Input: part model. Units: mm. Frame: model coordinates. Coordinates: 2 decimals unless noted, no trailing zeros. Loops run counter-clockwise (first coordinate to the right, second up) from the corner with the lowest first, then second, coordinate; pieces in that order, holes last. Notation, with made-up numbers: (16.25, -15.5) - (26.25, -15.5) arc R21 cw to (26.25, 15.5) - close; hole circle Ø11 at (-15, -26.75). An arc over 180 degrees is marked (long way). Use a Markdown table: item, result. Add a question column.
1. Section query D-D on x = 40. Return the cut outline in (y, z), then the cut area to 3 significant figures.
2. Section query A-A on z = 12.25. Return the cut outline in (x, y), then the cut area to 3 significant figures.
3. Ray query, L1, parallel to X at y = 1, z = 11.5; L2, parallel to X at y = 0.8, z = 4; L3, parallel to X at y = 0.85, z = 6.5. Return the intervals inside material, ascending. Write a range as [from, to].
4. Contact query for a flat-ended pin moving along its axis: P1, Ø1, axis at x = 44.5, z = 7, coming from the +Y side. Output: stop coordinate, or through.
5. Draft query along X for faces 1 (the face through (30, 0, 8)), 2 (the face through (23.2, 1.5, 7.5)), 3 (the face through (46.4, 1.5, 7.5)), 4 (the face through (-4.866, 2, 9)). Return one class per face: released by +X, released by -X, zero draft, split by the parting line, or undercut.
6. Section query C-C on z = 4. Return the cut outline in (x, y), then the cut area to 3 significant figures.
7. Section query B-B on y = 2. Return the cut outline in (x, z) (3 decimals), then the cut area to 3 significant figures.
```python
from build123d import *

# Parameters (mm, degrees)
BOSS_EXTRUDE1_DEPTH = 3
SKETCH2_W           = 75.494873271
SKETCH2_H           = 16.574066579
CUT_EXTRUDE1_DEPTH  = 3
FILLET1_R           = 0.5


with BuildPart() as part:
    # Sketch1 → Boss-Extrude1 (new body)
    with BuildSketch(Plane(origin=(0, 0, 0), x_dir=(1, 0, 0), z_dir=(0, 1, 0))):
        with BuildLine():
            ThreePointArc((51.666035076, -4.495071474), (57.875, -2.537392354), (64.083964924, -4.495071474))
            Line((64.083964924, -4.495071474), (64.083964924, -11.181167218))
            ThreePointArc((64.083964924, -11.181167218), (57.875, -9.223488098), (51.666035076, -11.181167218))
            ThreePointArc((51.666035076, -11.181167218), (46.3, -13.686095744), (40.933964924, -11.181167218))
            ThreePointArc((40.933964924, -11.181167218), (34.725, -9.223488098), (28.516035077, -11.181167218))
            ThreePointArc((28.516035077, -11.181167218), (23.15, -13.686095744), (17.783964924, -11.181167218))
            ThreePointArc((17.783964924, -11.181167218), (11.575, -9.223488098), (5.366035077, -11.181167218))
            ThreePointArc((5.366035077, -11.181167218), (0, -13.686095744), (-5.366035076, -11.181167218))
            Line((-5.366035076, -11.181167218), (-5.366035076, -4.495071474))
            ThreePointArc((-5.366035076, -4.495071474), (0, -7), (5.366035076, -4.495071474))
            ThreePointArc((5.366035076, -4.495071474), (11.575, -2.537392354), (17.783964924, -4.495071474))
            ThreePointArc((17.783964924, -4.495071474), (23.15, -7), (28.516035076, -4.495071474))
            ThreePointArc((28.516035076, -4.495071474), (34.725, -2.537392354), (40.933964924, -4.495071474))
            ThreePointArc((40.933964924, -4.495071474), (46.3, -7), (51.666035076, -4.495071474))
        make_face()
    extrude(amount=BOSS_EXTRUDE1_DEPTH)

    # Sketch2 → Cut-Extrude1 (cut)
    with BuildSketch(Plane(origin=(0, 3, 0), x_dir=(1, 0, 0), z_dir=(0, 1, 0))):
        with Locations((29.270514079, -6.984979931)):
            Rectangle(SKETCH2_W, SKETCH2_H)
        with BuildLine():
            Line((63.583964924, -10.267724094), (63.583964924, -4.759291488))
            ThreePointArc((63.583964924, -4.759291488), (57.778030808, -3.037847716), (52.005454008, -4.868038061))
            ThreePointArc((52.005454008, -4.868038061), (46.3, -7.5), (40.594545992, -4.868038061))
            ThreePointArc((40.594545992, -4.868038061), (34.725, -3.037392354), (28.855454008, -4.868038061))
            ThreePointArc((28.855454008, -4.868038061), (23.15, -7.5), (17.444545992, -4.868038061))
            ThreePointArc((17.444545992, -4.868038061), (11.575, -3.037392354), (5.705454008, -4.868038061))
            ThreePointArc((5.705454008, -4.868038061), (0.593454673, -7.476483903), (-4.866035076, -5.707162398))
            Line((-4.866035076, -5.707162398), (-4.866035076, -10.995585579))
            ThreePointArc((-4.866035076, -10.995585579), (0.121449449, -13.184961032), (5.023650974, -10.810769172))
            ThreePointArc((5.023650974, -10.810769172), (11.575, -8.723488098), (18.126349026, -10.810769172))
            ThreePointArc((18.126349026, -10.810769172), (23.15, -13.186095744), (28.173650974, -10.810769172))
            ThreePointArc((28.173650974, -10.810769172), (34.725, -8.723488098), (41.276349026, -10.810769172))
            ThreePointArc((41.276349026, -10.810769172), (46.3, -13.186095744), (51.323650974, -10.810769172))
            ThreePointArc((51.323650974, -10.810769172), (57.373874034, -8.734580825), (63.583964924, -10.267724094))
        make_face(mode=Mode.SUBTRACT)
    extrude(amount=-CUT_EXTRUDE1_DEPTH, mode=Mode.SUBTRACT)

    # Fillet1
    fillet1_edges = [part.edges().sort_by_distance(p)[0] for p in [
        (63.583964924, 1.5, 10.267724094),
        (63.583964924, 1.5, 4.759291488),
        (-4.866035076, 1.5, 5.707162398),
        (-4.866035076, 1.5, 10.995585579),
    ]]
    fillet(fillet1_edges, radius=FILLET1_R)


solid = part.part
```
Resolved:
| question | item | result |
|---|---|---|
| 1 | outline | (0, 4.49) - (3, 4.49) - (3, 10.03) - (0, 10.03) - close |
| 1 | area | 16.6 mm² |
| 2 | outline | (-3.36, 0) - (3.36, 0) - (3.36, 3) - (-3.36, 3) - close; (19.79, 0) - (26.51, 0) - (26.51, 3) - (19.79, 3) - close; (42.94, 0) - (49.66, 0) - (49.66, 3) - (42.94, 3) - close |
| 2 | area | 60.5 mm² |
| 3 | L1 | [-4.37, 4.37], [18.78, 27.52], [41.93, 50.67] |
| 3 | L2 | [7.22, 15.93], [30.37, 39.08], [53.52, 62.23] |
| 3 | L3 | [-4.82, -3.74], [3.74, 19.41], [26.89, 42.56], [50.04, 63.58] |
| 4 | P1 | y = 3 |
| 5 | face 1 | zero draft |
| 5 | face 2 | undercut |
| 5 | face 3 | undercut |
| 5 | face 4 | released by -X |
| 6 | outline | (7.22, 0) - (15.93, 0) - (15.93, 3) - (7.22, 3) - close; (30.37, 0) - (39.08, 0) - (39.08, 3) - (30.37, 3) - close; (53.52, 0) - (62.23, 0) - (62.23, 3) - (53.52, 3) - close |
| 6 | area | 78.4 mm² |
| 7 | outline | (-4.866, 6.704) arc R0.5 ccw to (-4.093, 6.285) arc R7.5 cw to (5.705, 4.868) arc R10.325 ccw to (17.445, 4.868) arc R7.5 cw to (28.855, 4.868) arc R10.325 ccw to (40.595, 4.868) arc R7.5 cw to (52.005, 4.868) arc R10.325 ccw to (63.349, 4.608) arc R0.5 ccw to (63.584, 5.032) - (63.584, 9.433) arc R0.5 ccw to (62.864, 9.881) arc R11.325 cw to (51.324, 10.811) arc R6.5 ccw to (41.276, 10.811) arc R11.325 cw to (28.174, 10.811) arc R6.5 ccw to (18.126, 10.811) arc R11.325 cw to (5.024, 10.811) arc R6.5 ccw to (-4.73, 11.145) arc R0.5 ccw to (-4.866, 10.802) - close |
| 7 | area | 382 mm² |
